For this review, take the finished solid that the model builds, in its own axes (mm). Give positions to 0.01 mm unless a question says otherwise; leave off trailing zeros. Write each loop counter-clockwise with the first axis right and the second up, starting at its lowest first coordinate (ties: lowest second). Pieces come first, ordered by that corner, then holes.
Q1. For line 1 (Z direction, x = -17.5, y = 0.75); line 2 (Z direction, x = -111, y = -5.25); line 3 (X direction, y = -5, z = 25.5), list the stretches that pass through material, from the lowest coordinate up.
Q2. Insertion check: P1, Ø12, axis at x = -40.5, z = 38.5, coming from the +Y side; P2, Ø0.9, axis at y = 1, z = 36, coming from the -X side (3 decimals); P3, Ø1.5, axis at x = -175.5, z = 36.5, coming from the -Y side. Each pin has a flat end and moves straight along its axis. Give the tip position at first contact, or say it passes through.
Q3. We need section B-B (z = 13). Write out the cut boundary in (x, y) (3 decimals), then the cut area to 3 significant figures.
Q4. We need section A-A (x = -176). Write out the cut boundary in (y, z), then the cut area to 3 significant figures.
Q5. We need section D-D (x = -71). Write out the cut boundary in (y, z).
Q6. We need section C-C (y = -2). Write out the cut boundary in (x, z) (3 decimals).
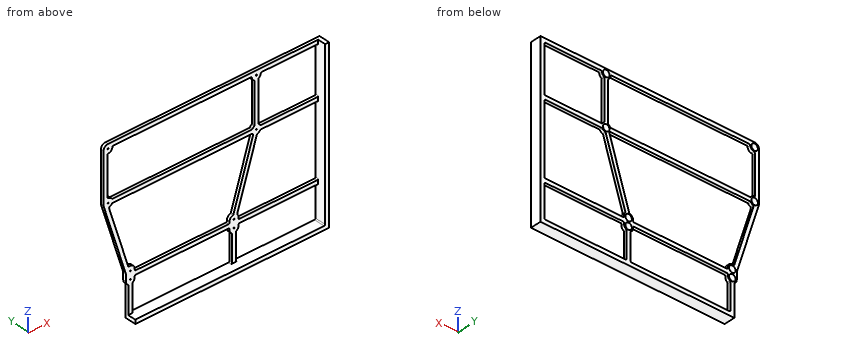
```python
from build123d import *

# Parameters (mm, degrees)
SKETCH1_R           = 0.5
BOSS_EXTRUDE1_DEPTH = 3
BOSS_EXTRUDE2_DEPTH = 8
CHAMFER1_SIZE       = 2.8
FILLET1_R           = 1


with BuildPart() as part:
    # Sketch1 → Boss-Extrude1 (new body)
    with BuildSketch(Plane(origin=(0, 0, 0), x_dir=(1, 0, 0), z_dir=(0, 1, 0))):
        with BuildLine():
            Line((-191.955, 0), (-191.955, 4))
            Line((-191.955, 4), (4, 4))
            Line((4, 4), (4, -167))
            Line((4, -167), (0, -167))
            Line((0, -167), (-212.5, -167))
            ThreePointArc((-212.5, -167), (-215.681980515, -165.681980515), (-217, -162.5))
            Line((-217, -162.5), (-217, -112.5))
            ThreePointArc((-217, -112.5), (-216.949028292, -111.824613255), (-216.797267886, -111.164526783))
            Line((-216.797267886, -111.164526783), (-194.455, -39.271875472))
            Line((-194.455, -39.271875472), (-194.455, -32.045))
            ThreePointArc((-194.455, -32.045), (-193.779264635, -29.673291755), (-191.955, -28.013871126))
            Line((-191.955, -28.013871126), (-191.955, 0))
        make_face()
        with Locations((-62.5, -162.5)):
            Circle(SKETCH1_R, mode=Mode.SUBTRACT)
        with Locations((-62.5, -112.5)):
            Circle(SKETCH1_R, mode=Mode.SUBTRACT)
        with Locations((-212.5, -112.5)):
            Circle(SKETCH1_R, mode=Mode.SUBTRACT)
        with Locations((-212.5, -162.5)):
            Circle(SKETCH1_R, mode=Mode.SUBTRACT)
        with Locations((-189.955, -32.045)):
            Circle(SKETCH1_R, mode=Mode.SUBTRACT)
        with Locations((-189.955, -39.955)):
            Circle(SKETCH1_R, mode=Mode.SUBTRACT)
        with Locations((-85.045, -32.045)):
            Circle(SKETCH1_R, mode=Mode.SUBTRACT)
        with Locations((-85.045, -39.955)):
            Circle(SKETCH1_R, mode=Mode.SUBTRACT)
        with BuildLine():
            Line((0, 0), (-83.045, 0))
            Line((-83.045, 0), (-83.045, -28.013871126))
            ThreePointArc((-83.045, -28.013871126), (-81.220735365, -29.673291755), (-80.545, -32.045))
            Line((-80.545, -32.045), (-80.545, -34))
            Line((-80.545, -34), (0, -34))
            Line((0, -34), (0, 0))
        make_face(mode=Mode.SUBTRACT)
        with BuildLine():
            Line((0, -163), (0, -114.5))
            Line((0, -114.5), (-58.468871126, -114.5))
            ThreePointArc((-58.468871126, -114.5), (-59.318019485, -115.681980515), (-60.5, -116.531128874))
            Line((-60.5, -116.531128874), (-60.5, -158.468871126))
            ThreePointArc((-60.5, -158.468871126), (-58.549693914, -160.344754811), (-58.027864045, -163))
            Line((-58.027864045, -163), (0, -163))
        make_face(mode=Mode.SUBTRACT)
        with BuildLine():
            Line((-185.455, -32.045), (-185.455, -34))
            Line((-185.455, -34), (-89.545, -34))
            Line((-89.545, -34), (-89.545, -32.045))
            ThreePointArc((-89.545, -32.045), (-88.869264635, -29.673291755), (-87.045, -28.013871126))
            Line((-87.045, -28.013871126), (-87.045, 0))
            Line((-87.045, 0), (-187.955, 0))
            Line((-187.955, 0), (-187.955, -28.013871126))
            ThreePointArc((-187.955, -28.013871126), (-186.130735365, -29.673291755), (-185.455, -32.045))
        make_face(mode=Mode.SUBTRACT)
        with BuildLine():
            Line((-58.468871126, -110.5), (0, -110.5))
            Line((0, -110.5), (0, -38))
            Line((0, -38), (-80.545, -38))
            Line((-80.545, -38), (-80.545, -39.955))
            ThreePointArc((-80.545, -39.955), (-80.908092918, -41.725875431), (-81.938777685, -43.210976494))
            Line((-81.938777685, -43.210976494), (-61.786428638, -108.056936202))
            ThreePointArc((-61.786428638, -108.056936202), (-59.831632472, -108.876491377), (-58.468871126, -110.5))
        make_face(mode=Mode.SUBTRACT)
        with BuildLine():
            Line((-208.027864045, -163), (-66.972135955, -163))
            ThreePointArc((-66.972135955, -163), (-66.450306086, -160.344754811), (-64.5, -158.468871126))
            Line((-64.5, -158.468871126), (-64.5, -116.531128874))
            ThreePointArc((-64.5, -116.531128874), (-65.681980515, -115.681980515), (-66.531128874, -114.5))
            Line((-66.531128874, -114.5), (-208.468871126, -114.5))
            ThreePointArc((-208.468871126, -114.5), (-210.344754811, -116.450306086), (-213, -116.972135955))
            Line((-213, -116.972135955), (-213, -158.027864045))
            ThreePointArc((-213, -158.027864045), (-209.318019485, -159.318019485), (-208.027864045, -163))
        make_face(mode=Mode.SUBTRACT)
        with BuildLine():
            Line((-191.759678163, -44.077273248), (-211.650270256, -108.080954926))
            ThreePointArc((-211.650270256, -108.080954926), (-209.776281957, -108.917911221), (-208.468871126, -110.5))
            Line((-208.468871126, -110.5), (-66.531128874, -110.5))
            ThreePointArc((-66.531128874, -110.5), (-66.123508623, -109.831632472), (-65.606222315, -109.244023506))
            Line((-65.606222315, -109.244023506), (-85.758571362, -44.398063798))
            ThreePointArc((-85.758571362, -44.398063798), (-88.469986944, -42.873812162), (-89.545, -39.955))
            Line((-89.545, -39.955), (-89.545, -38))
            Line((-89.545, -38), (-185.455, -38))
            Line((-185.455, -38), (-185.455, -39.955))
            ThreePointArc((-185.455, -39.955), (-187.492384696, -43.721367728), (-191.759678163, -44.077273248))
        make_face(mode=Mode.SUBTRACT)
    extrude(amount=BOSS_EXTRUDE1_DEPTH)

    # Sketch2 → Boss-Extrude2 (add)
    with BuildSketch(Plane.XZ):
        Polygon((4, -4), (4, 167), (0, 167), (0, 0), (-191.955, 0), (-191.955, -4), align=None)
    extrude(amount=BOSS_EXTRUDE2_DEPTH)

    # Chamfer1
    chamfer1_edges = [part.edges().sort_by_distance(p)[0] for p in [
        (-63, 3, 112.5),
        (-213, 3, 112.5),
        (-213, 3, 162.5),
        (-63, 3, 162.5),
        (-190.455, 3, 32.045),
        (-190.455, 3, 39.955),
        (-85.545, 3, 32.045),
        (-85.545, 3, 39.955),
    ]]
    chamfer(chamfer1_edges, length=CHAMFER1_SIZE)

    # Fillet1
    fillet1_edges = [part.edges().sort_by_distance(p)[0] for p in [
        (-89.545, 1.5, 34),
        (-87.045, 1.5, 28.013871126),
        (-87.045, 1.5, 0),
        (-187.955, 1.5, 0),
        (-191.759678163, 1.5, 44.077273248),
        (-211.650270256, 1.5, 108.080954926),
        (-208.468871126, 1.5, 110.5),
        (-66.531128874, 1.5, 110.5),
        (-65.606222315, 1.5, 109.244023506),
        (-85.758571362, 1.5, 44.398063798),
        (-89.545, 1.5, 38),
        (-185.455, 1.5, 38),
        (-81.938777685, 1.5, 43.210976494),
        (-61.786428638, 1.5, 108.056936202),
        (-58.468871126, 1.5, 110.5),
        (0, 1.5, 110.5),
        (0, 1.5, 38),
        (-80.545, 1.5, 38),
        (-194.455, 1.5, 39.271875472),
        (-191.955, 1.5, 28.013871126),
        (0, 1.5, 34),
        (0, -2.5, 0),
        (-83.045, 1.5, 0),
        (-83.045, 1.5, 28.013871126),
        (-80.545, 1.5, 34),
        (-66.972135955, 1.5, 163),
        (-64.5, 1.5, 158.468871126),
        (-64.5, 1.5, 116.531128874),
        (-66.531128874, 1.5, 114.5),
        (-208.468871126, 1.5, 114.5),
        (-213, 1.5, 116.972135955),
        (-213, 1.5, 158.027864045),
        (-208.027864045, 1.5, 163),
        (-60.5, 1.5, 158.468871126),
        (-58.027864045, 1.5, 163),
        (0, 1.5, 163),
        (0, 1.5, 114.5),
        (-58.468871126, 1.5, 114.5),
        (-60.5, 1.5, 116.531128874),
        (-187.955, 1.5, 28.013871126),
        (-185.455, 1.5, 34),
    ]]
    fillet(fillet1_edges, radius=FILLET1_R)


solid = part.part
```
Computed:
1. line 1: z = -4 to 0, 34 to 38, 110.5 to 114.5, 163 to 167
1. line 2: z = -4 to 0
1. line 3: x = 0 to 4
2. P1: stops at y = 3
2. P2: stops at x = -194.455
2. P3: stops at y = 0
3. outline: (-191.955, 0) - (-187.955, 0) - (-187.955, 3) - (-191.955, 3) - close; (-87.045, 0) - (-83.045, 0) - (-83.045, 3) - (-87.045, 3) - close; (0, -8) - (4, -8) - (4, 3) - (0, 3) - close
3. area: 68.0 mm2
4. outline: (-8, -4) - (3, -4) - (3, 0) - (-8, 0) - close; (0, 34) - (3, 34) - (3, 38) - (0, 38) - close; (0, 110.5) - (3, 110.5) - (3, 114.5) - (0, 114.5) - close; (0, 163) - (3, 163) - (3, 167) - (0, 167) - close
4. area: 80.0 mm2
5. outline: (-8, -4) - (3, -4) - (3, 0) - (-8, 0) - close; (0, 34) - (3, 34) - (3, 38) - (0, 38) - close; (0, 78.41) - (3, 78.41) - (3, 91.89) - (0, 91.89) - close; (0, 110.5) - (3, 110.5) - (3, 114.5) - (0, 114.5) - close; (0, 163) - (3, 163) - (3, 167) - (0, 167) - close
6. outline: (-191.955, -4) - (4, -4) - (4, 167) - (0, 167) - (0, 1) arc R1 cw to (-1, 0) - (-191.955, 0) - close
